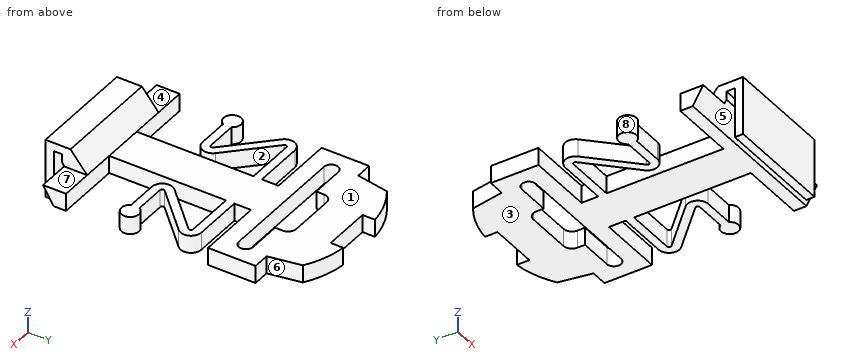
```python
from build123d import *

# Parameters (mm, degrees)
Y_KSEKLIK_EKSTR_ZYON2_DEPTH = 2.1
Y_KSEKLIK_EKSTR_ZYON3_DEPTH = 10.35
KES_EKSTR_ZYON1_DEPTH       = 36.16052474
KES_EKSTR_ZYON2_DEPTH       = 3.85


with BuildPart() as part:
    # Çizim1 → Yükseklik-Ekstrüzyon2 (new body)
    with BuildSketch(Plane.XY):
        with BuildLine():
            Line((0, 0), (-10.35, 0))
            Line((-10.35, 0), (-10.35, 5))
            Line((-10.35, 5), (-2.5, 5))
            Line((-2.5, 5), (-2.5, 19))
            Line((-2.5, 19), (-8.5, 19))
            ThreePointArc((-8.5, 19), (-8.730969883, 18.845670858), (-8.676776695, 18.573223305))
            Line((-8.676776695, 18.573223305), (-3.737436867, 13.633883476))
            ThreePointArc((-3.737436867, 13.633883476), (-3.466470928, 12.27164571), (-4.621320344, 11.5))
            Line((-4.621320344, 11.5), (-8.376690734, 11.5))
            ThreePointArc((-8.376690734, 11.5), (-10.35, 12), (-8.376690734, 12.5))
            Line((-8.376690734, 12.5), (-4.621320344, 12.5))
            ThreePointArc((-4.621320344, 12.5), (-4.39035046, 12.654329142), (-4.444543648, 12.926776695))
            Line((-4.444543648, 12.926776695), (-9.383883476, 17.866116524))
            ThreePointArc((-9.383883476, 17.866116524), (-9.654849416, 19.22835429), (-8.5, 20))
            Line((-8.5, 20), (-2.5, 20))
            Line((-2.5, 20), (-2.5, 22))
            Line((-2.5, 22), (-10.35, 22))
            Line((-10.35, 22), (-10.35, 27.7))
            Line((-10.35, 27.7), (-8.35, 27.7))
            Line((-8.35, 27.7), (-7.662324775, 31.6))
            ThreePointArc((-7.662324775, 31.6), (-5.382058591, 32.732647346), (-2.9, 33.3))
            Line((-2.9, 33.3), (-2.9, 31.8))
            Line((-2.9, 31.8), (0, 31.8))
            Line((0, 31.8), (0, 27.6))
            Line((0, 27.6), (-2.75, 27.6))
            ThreePointArc((-2.75, 27.6), (-3.457106781, 27.307106781), (-3.75, 26.6))
            Line((-3.75, 26.6), (-3.75, 25.7))
            Line((-3.75, 25.7), (-7.75, 25.7))
            ThreePointArc((-7.75, 25.7), (-8.6, 24.85), (-7.75, 24))
            Line((-7.75, 24), (0, 24))
            Line((0, 24), (0, 0))
        make_face()
    extrude(amount=Y_KSEKLIK_EKSTR_ZYON2_DEPTH)

    # Çizim2 → Yükseklik-Ekstrüzyon3 (add, through all)
    with BuildSketch(Plane(origin=(0, 0, 0), x_dir=(0, 0, -1), z_dir=(1, 0, 0))):
        Polygon((0, 5), (0, 3.5), (-2.5, 2), (-3.5, 2), (-3.5, 1), (2.5, 1), (2.5, 0), (-4.5, 0), (-4.5, 3), (-2.1, 5), align=None)
    extrude(amount=-Y_KSEKLIK_EKSTR_ZYON3_DEPTH)

    # Çizim2<3> → Kes-Ekstrüzyon1 (cut, through all)
    with BuildSketch(Plane(origin=(0, 0, 0), x_dir=(0, 0, -1), z_dir=(1, 0, 0))):
        Polygon((0, 3.5), (2.5, 1), (-3.5, 1), (-3.5, 2), (-2.5, 2), align=None)
    extrude(amount=-KES_EKSTR_ZYON1_DEPTH, mode=Mode.SUBTRACT)

    # Çizim3 → Kes-Ekstrüzyon2 (cut)
    with BuildSketch(Plane.ZY.offset(10.35)):
        Polygon((4.5, 3), (2.1, 5), (2.1, 2.24), (2.5, 2), (3.5, 2), (3.5, 1), (-2.5, 1), (-2.5, 0), (4.5, 0), align=None)
    extrude(amount=-KES_EKSTR_ZYON2_DEPTH, mode=Mode.SUBTRACT)

    # Aynalama1: part across plane


with BuildPart() as part_1:
    add(part.part)
    add(part.part.mirror(Plane(origin=(0, 24, 2.1), x_dir=(0, 0, 1), z_dir=(1, 0, 0))))


solid = part_1.part
```
Source: CAD feature listing. Evaluate the final solid. Frame: model axes, mm. Face numbers are marked on the shaded views. A direction names the side the tool comes from. Coordinates: 2 decimals unless noted, no trailing zeros. Order: outer loops, then holes, each group sorted by start corner. A loop starts at its lowest first (then second) coordinate and runs counter-clockwise, first axis right, second up. Notation, with made-up numbers: (-2.5, 56.25) - (27.5, 56.25) arc R24 ccw to (27.5, 86.25) - close; hole circle Ø10 at (5, -14). An arc over 180 degrees is marked (long way). One line per item, written item: value.
1) Mould query, pull axis X, two halves, no side actions, for the marked faces 6, 7 and 8. Classes: released by +X, released by -X, zero draft, split by the parting line, or undercut.
Computed values:
face 6: released by +X
face 7: zero draft
face 8: undercut
2) Contact query for flat-ended pins moving along their axis: pin 1 (2.5 mm diameter, centred on x = -7, z = 1, fed in from +Y); pin 2 (1.7 mm diameter, centred on x = -4.5, z = 1, fed in from -Y); pin 3 (4 mm diameter, centred on x = -2, y = 12, fed in from +Z); pin 4 (1.5 mm diameter, centred on y = 9, z = -1.5, fed in from -X). Output: stop coordinate, or through.
Computed values:
pin 1: stops at y = 32.59
pin 2: stops at y = 0
pin 3: stops at z = 2.1
pin 4: passes through
3) Cut plane A-A on y = 24.85. Output: boundary loops of the cut face in (x, z).
Computed values:
outline: (-10.35, 0) - (-8.6, 0) - (-8.6, 2.1) - (-10.35, 2.1) - close; (8.6, 0) - (10.35, 0) - (10.35, 2.1) - (8.6, 2.1) - close
4) Ray query, line 1 (Y direction, x = 0.75, z = 1.25); line 2 (Y direction, x = 2.75, z = 1); line 3 (Y direction, x = -3, z = 2). Return the intervals inside material, ascending. Write a range as [from, to].
Computed values:
line 1: y = [0, 1], [2.75, 24], [27.6, 31.8]
line 2: y = [0, 1], [2.9, 5], [19, 20], [22, 24], [27.6, 31.8]
line 3: y = [0, 1], [2.3, 5], [19, 20], [22, 24], [27.57, 33.29]
5) Cut plane C-C on z = 1. State how many separate pieces and enclosed holes the cut face has, plus the area to 3 significant figures.
Computed values:
separate pieces: 2
enclosed holes: 1
area: 338 mm^2
6) Cut plane B-B on x = -0.5. Output: boundary loops of the cut face in (y, z), plus the area to 3 significant figures.
Computed values:
outline: (0, -2.5) - (1, -2.5) - (1, 3.5) - (2, 3.5) - (2, 2.5) - (3.5, 0) - (24, 0) - (24, 2.1) - (5, 2.1) - (3, 4.5) - (0, 4.5) - close; (27.6, 0) - (31.8, 0) - (31.8, 2.1) - (27.6, 2.1) - close
area: 65.9 mm^2
7) Reachability of the marked faces 1, 2, 3, 4 and 5 from +Z, -Z, +X, -X, +Y, -Y: full face, straight path, thin tool, end or side. Return the list, or none.
Computed values:
face 1: +Z, +X, -X, +Y
face 2: +Z, -Z
face 3: -Z, +X, -X, +Y
face 4: +Z, -X, +Y, -Y
face 5: -Z, +X, -X
